Could you check a few things on this drawing? It's one solid part, dimensions in mm from its lowest x, y, z. A direction names the side the tool comes from. Round coordinates to 2 decimals unless told otherwise and drop trailing zeros. Order: outer loops, then holes, each group sorted by start corner. A loop starts at its lowest first (then second) coordinate and runs counter-clockwise, first axis right, second up.
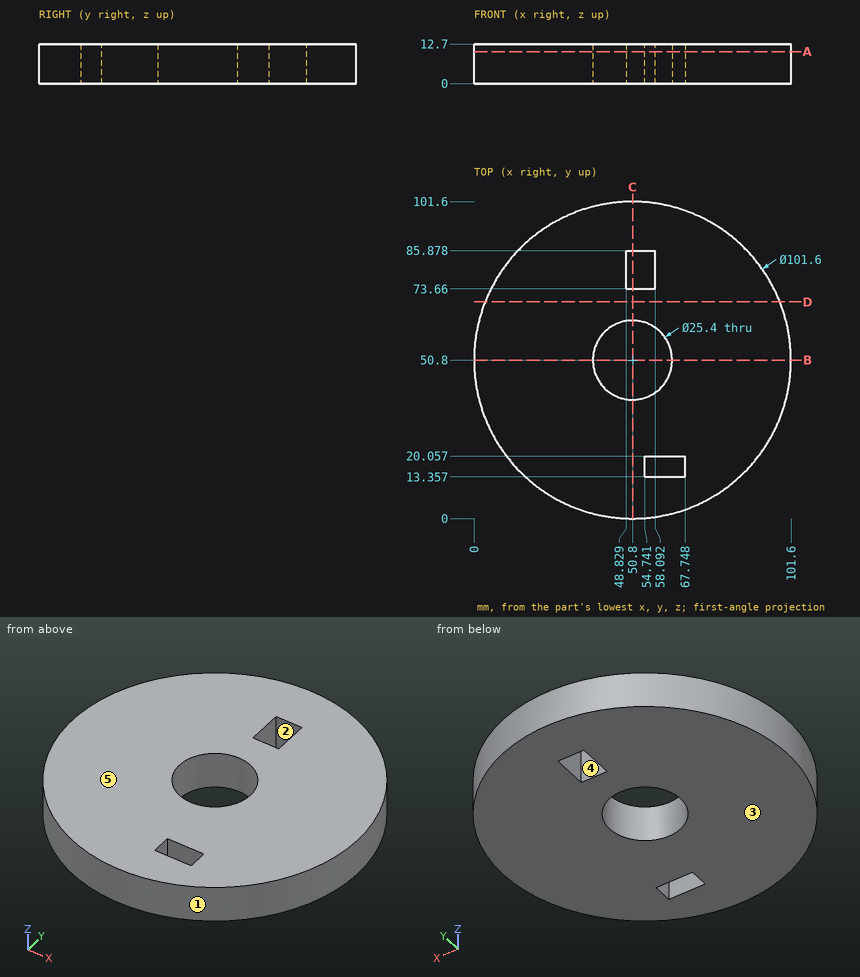
(1) I want a section at B-B, the plane y = 50.8. List the corners of the cut face in (x, z) for me.
(2) If we mould it in two halves opening along Y, with no side actions, what happens to the marked faces 1, 2 and 3? For each: pulls with the +Y half, pulls with the -Y half, needs draft (parallel to the pull), parting line crosses it, or undercut.
(3) I want a section at C-C, the plane x = 50.8. List the corners of the cut face in (y, z) for me.
(4) Please list where these lines run through material, in increasing order: probe 1 along Y at (x, z) = (50.8, 3.25); probe 2 along X at (y, z) = (43, 7.25); probe 3 along X at (y, z) = (77.5, 10.25).
(5) On a 3-axis mill with a long thin cutter (end or side, diameter ignored), from which of +Z, -Z, +X, -X, +Y, -Y can I reach the whole of each face in a straight line? I mean the marked faces 4 and 5. Say none if no direction works.
(6) I want a section at A-A, the plane z = 10.25. List the corners of the cut face in (x, y) for me.
(7) I'm going to push flat-ended pins straight in: pin 1 Ø4 at (x, z) = (59.5, 6.5) entering from +Y; pin 2 Ø2 at (y, z) = (17.5, 5.5) entering from +X; pin 3 Ø4.5 at (x, z) = (55, 6.5) entering from +Y. Where does each tip first touch, or does it pass through?
(8) I want a section at D-D, the plane y = 69.5. List the corners of the cut face in (x, z) for me, plus the area to 3 significant figures.
Ans:
1. outline: (0, 0) - (38.1, 0) - (38.1, 12.7) - (0, 12.7) - close; (63.5, 0) - (101.6, 0) - (101.6, 12.7) - (63.5, 12.7) - close
2. face 1: parting line crosses it
2. face 2: undercut
2. face 3: needs draft
3. outline: (0, 0) - (38.1, 0) - (38.1, 12.7) - (0, 12.7) - close; (63.5, 0) - (73.66, 0) - (73.66, 12.7) - (63.5, 12.7) - close; (85.88, 0) - (101.6, 0) - (101.6, 12.7) - (85.88, 12.7) - close
4. probe 1: y = 0 to 38.1, 63.5 to 73.66, 85.88 to 101.6
4. probe 2: x = 0.6 to 40.78, 60.82 to 101
4. probe 3: x = 7.58 to 48.83, 58.09 to 94.02
5. face 4: +Z, -Z
5. face 5: +Z, +X, -X, +Y, -Y
6. outline: circle Ø101.6 at (50.8, 50.8); hole circle Ø25.4 at (50.8, 50.8); hole (48.83, 73.66) - (58.09, 73.66) - (58.09, 85.88) - (48.83, 85.88) - close; hole (54.74, 13.36) - (67.75, 13.36) - (67.75, 20.06) - (54.74, 20.06) - close
7. pin 1: stops at y = 101.16
7. pin 2: stops at x = 90.01
7. pin 3: stops at y = 101.56
8. outline: (3.57, 0) - (98.03, 0) - (98.03, 12.7) - (3.57, 12.7) - close
8. area: 1,200 mm2
